Read the model definition and answer for the solid it produces. Units are mm, in the model's axes. A direction names the side the tool comes from. Give positions to 0.01 mm unless a question says otherwise; leave off trailing zeros. Loops run counter-clockwise (first coordinate to the right, second up) from the corner with the lowest first, then second, coordinate; pieces in that order, holes last. Notation, with made-up numbers: (75.5, -32) - (116.5, -32) arc R29 ccw to (116.5, -8) - close; hole circle Ø7 at (87.25, 64.5). An arc over 180 degrees is marked (long way). Use a Markdown table: item, result. Add a question column.
Item 1: Consider probe 1 along Y at (x, z) = (-20, -3.75); probe 2 along X at (y, z) = (-23.5, 10.5); probe 3 along Z at (x, y) = (18, -11). Determine where each line is inside the solid, lowest interval first. Write a range as [from, to].
Item 2: A cutting plane is placed at B-B (x = -36). Determine the outline of the cut face in (y, z), plus the area to 3 significant figures.
Item 3: This flat-tipped pin is pushed along its axis until it touches: P1, Ø1.5, axis at x = 3, y = -1, coming from the +Z side. Where does it stop, or does it pass through?
Item 4: A cutting plane is placed at D-D (y = 4.5). Determine the outline of the cut face in (x, z), plus the area to 3 significant figures.
Item 5: Which of the six approach directions +Z, -Z, +X, -X, +Y, -Y give full straight-line access (tool end or side, diameter ignored) to faces 1 (the face through (44, -6.163, 0)), 2 (the face through (-1, -1, -12.7)), 3 (the face through (-1, 0, -10.16))?
Item 6: For a pull along Y with two mould halves and no side action, classify faces 4 (the face through (-4, 37, 12.7)), 5 (the face through (-1, 38.1, 0)), 6 (the face through (44, -14, 4.128)) as +Y half, -Y half, draft (parallel to the pull), parting line (faces both ways), or undercut.
Item 7: A cutting plane is placed at A-A (z = 0). Determine the outline of the cut face in (x, y), plus the area to 3 significant figures.
Item 8: A cutting plane is placed at C-C (z = 9.5). Determine the outline of the cut face in (x, y).
from build123d import *

# Parameters (mm, degrees)
F0_W     = 91.44
F0_H     = 25.4
F1_DEPTH = 38.1
F2_T     = -2.54
F3_W     = 15.875
F3_H     = 8.255
F3_R     = 3.175
F4_DEPTH = 2.54


with BuildPart() as f1:
    # F0 (on Front) → F1 (new body, symmetric)
    with BuildSketch(Plane.XZ):
        Rectangle(F0_W, F0_H)
    extrude(amount=F1_DEPTH, both=True)

    # F2
    f2_openings = [f1.faces().sort_by_distance(p)[0] for p in [
        (0, 0, 12.7),
    ]]
    offset(amount=F2_T, openings=f2_openings)

    # F3 (on face) → F4 (cut, through all)
    with BuildSketch(Plane.YZ.offset(45.72)):
        with Locations((-14.100978, 0)):
            Rectangle(F3_W, F3_H)
        with Locations((18.487949, 0)):
            Circle(F3_R)
    extrude(amount=-F4_DEPTH, mode=Mode.SUBTRACT)


solid = f1.part
Geometry says:
| question | item | result |
|---|---|---|
| 1 | probe 1 | [-38.1, -35.56], [35.56, 38.1] |
| 1 | probe 2 | [-45.72, -43.18], [43.18, 45.72] |
| 1 | probe 3 | [-12.7, -10.16] |
| 2 | outline | (-38.1, -12.7) - (38.1, -12.7) - (38.1, 12.7) - (35.56, 12.7) - (35.56, -10.16) - (-35.56, -10.16) - (-35.56, 12.7) - (-38.1, 12.7) - close |
| 2 | area | 310 mm² |
| 3 | P1 | z = -10.16 |
| 4 | outline | (-45.72, -12.7) - (45.72, -12.7) - (45.72, 12.7) - (43.18, 12.7) - (43.18, -10.16) - (-43.18, -10.16) - (-43.18, 12.7) - (-45.72, 12.7) - close |
| 4 | area | 348 mm² |
| 5 | face 1 | +X |
| 5 | face 2 | -Z, +X, -X, +Y, -Y |
| 5 | face 3 | +Z |
| 6 | face 4 | draft |
| 6 | face 5 | +Y half |
| 6 | face 6 | undercut |
| 7 | outline | (-45.72, -38.1) - (45.72, -38.1) - (45.72, -22.04) - (43.18, -22.04) - (43.18, -35.56) - (-43.18, -35.56) - (-43.18, 35.56) - (43.18, 35.56) - (43.18, 21.66) - (45.72, 21.66) - (45.72, 38.1) - (-45.72, 38.1) - close; (43.18, -6.16) - (45.72, -6.16) - (45.72, 15.31) - (43.18, 15.31) - close |
| 7 | area | 769 mm² |
| 8 | outline | (-45.72, -38.1) - (45.72, -38.1) - (45.72, 38.1) - (-45.72, 38.1) - close; hole (-43.18, -35.56) - (43.18, -35.56) - (43.18, 35.56) - (-43.18, 35.56) - close |
